Input: part model. Units: mm. Frame: model coordinates. A direction names the side the tool comes from. Coordinates: 2 decimals unless noted, no trailing zeros. Order: outer loops, then holes, each group sorted by start corner. A loop starts at its lowest first (then second) coordinate and runs counter-clockwise, first axis right, second up. Notation, with made-up numbers: (-22, -29.75) - (26, -29.75) arc R28 ccw to (26, 7.25) - close; hole circle Ø6 at (38.25, 55.25). An arc over 180 degrees is marked (long way). One line per question, with ' | ' between items. Start each with the question number.
```python
from build123d import *

# Parameters (mm, degrees)
SKETCH1_W           = 20.32
SKETCH1_H           = 40.64
BOSS_EXTRUDE1_DEPTH = 6.35


with BuildPart() as part:
    # Sketch1 → Boss-Extrude1 (new body)
    with BuildSketch(Plane.XY):
        Polygon((0, 0), (41.275, 0), (41.275, 63.5), (7.796819617, 63.5), align=None)
        with BuildLine():
            ThreePointArc((28.015, 5.4325), (29.765, 3.6825), (31.515, 5.4325))
            Line((31.515, 5.4325), (31.515, 7.4325))
            ThreePointArc((31.515, 7.4325), (29.765, 9.1825), (28.015, 7.4325))
            Line((28.015, 7.4325), (28.015, 5.4325))
        make_face(mode=Mode.SUBTRACT)
        with BuildLine():
            ThreePointArc((18.015, 5.4325), (19.765, 3.6825), (21.515, 5.4325))
            Line((21.515, 5.4325), (21.515, 7.4325))
            ThreePointArc((21.515, 7.4325), (19.765, 9.1825), (18.015, 7.4325))
            Line((18.015, 7.4325), (18.015, 5.4325))
        make_face(mode=Mode.SUBTRACT)
        with BuildLine():
            ThreePointArc((31.515, 57.4325), (29.765, 59.1825), (28.015, 57.4325))
            Line((28.015, 57.4325), (28.015, 55.4325))
            ThreePointArc((28.015, 55.4325), (29.765, 53.6825), (31.515, 55.4325))
            Line((31.515, 55.4325), (31.515, 57.4325))
        make_face(mode=Mode.SUBTRACT)
        with BuildLine():
            ThreePointArc((21.515, 57.4325), (19.765, 59.1825), (18.015, 57.4325))
            Line((18.015, 57.4325), (18.015, 55.4325))
            ThreePointArc((18.015, 55.4325), (19.765, 53.6825), (21.515, 55.4325))
            Line((21.515, 55.4325), (21.515, 57.4325))
        make_face(mode=Mode.SUBTRACT)
        with Locations((24.765, 31.4325)):
            Rectangle(SKETCH1_W, SKETCH1_H, mode=Mode.SUBTRACT)
    extrude(amount=BOSS_EXTRUDE1_DEPTH)


solid = part.part
```
(1) Section B-B (y = 21). Output: boundary loops of the cut face in (x, z) (3 decimals), then the cut area to 3 significant figures.
(2) Draft query along Y for faces 3 (the face through (20, 0, 3)), 4 (the face through (11, 32, 0)), 5 (the face through (14.605, 31, 3)), 6 (the face through (21.515, 6, 3)). Return one class per face: +Y half, -Y half, draft (parallel to the pull), parting line (faces both ways), or undercut.
(3) Section A-A (z = 1.5). State how many separate pieces and enclosed holes the cut face has, then the cut area to 3 significant figures.
(4) Section C-C (x = 15.5). Output: boundary loops of the cut face in (y, z).
(5) Section D-D (x = 5.5). Output: boundary loops of the cut face in (y, z), then the cut area to 3 significant figures.
(6) Pin query (flat end, axial travel): pin 1 (1 mm diameter, centred on y = 57, z = 4, fed in from -X); pin 2 (2 mm diameter, centred on y = 31, z = 1.5, fed in from -X); pin 3 (2 mm diameter, centred on x = 12, y = 40.5, fed in from -Z); pin 4 (1.9 mm diameter, centred on y = 32, z = 4.5, fed in from -X). Return the tip coordinate at first contact, or that it passes through.
(7) Reachability of faces 1 (the face through (25, 63.5, 3)), 2 (the face through (25, 51.752, 3)) from +Z, -Z, +X, -X, +Y, -Y: full face, straight path, thin tool, end or side. Return the list, or none.
(8) Material intervals for line 1 along Y through (x, z) = (24, 1.75); line 2 along X through (y, z) = (54, 1.25) (3 decimals); line 3 along Y through (x, z) = (28.5, 2.5), sorted ascending. Write a range as from..to.
Worked answers:
1) outline: (2.578, 0) - (14.605, 0) - (14.605, 6.35) - (2.578, 6.35) - close; (34.925, 0) - (41.275, 0) - (41.275, 6.35) - (34.925, 6.35) - close | area: 117 mm²
2) face 3: -Y half | face 4: draft | face 5: undercut | face 6: undercut
3) separate pieces: 1 | enclosed holes: 5 | area: 1,480 mm²
4) outline: (0, 0) - (11.11, 0) - (11.11, 6.35) - (0, 6.35) - close; (51.75, 0) - (63.5, 0) - (63.5, 6.35) - (51.75, 6.35) - close
5) outline: (0, 0) - (44.79, 0) - (44.79, 6.35) - (0, 6.35) - close | area: 284 mm²
6) pin 1: stops at x = 6.94 | pin 2: stops at x = 3.68 | pin 3: stops at z = 0 | pin 4: stops at x = 3.81
7) face 1: +Z, -Z, +X, -X, +Y | face 2: +Z, -Z
8) line 1: y = 0..11.11, 51.75..63.5 | line 2: x = 6.63..18.76, 20.77..28.76, 30.77..41.275 | line 3: y = 0..4.22, 8.64..11.11, 51.75..54.22, 58.64..63.5
